Source: CAD feature listing. Evaluate the final solid. Frame: model axes, mm. A direction names the side the tool comes from. Round coordinates to 2 decimals unless told otherwise and drop trailing zeros. Write each loop counter-clockwise with the first axis right and the second up, starting at its lowest first coordinate (ties: lowest second). Pieces come first, ordered by that corner, then holes.
```python
from build123d import *

# Parameters (mm, degrees)
SKETCH1_R               = 4.7625
BOSS_EXTRUDE1_DEPTH     = 5.08
SKETCH2_W               = 5.08
SKETCH2_H               = 4.445
SKETCH3_R               = 1.27
CUT_EXTRUDE1_DEPTH      = 1
CUT_EXTRUDE1_DEPTH_BACK = 11.16


with BuildPart() as part:
    # Sketch1 → Boss-Extrude1 (new body, symmetric)
    with BuildSketch(Plane.XY):
        Circle(SKETCH1_R)
    extrude(amount=BOSS_EXTRUDE1_DEPTH, both=True)

    # Sketch2 → Cut-Revolve1 (revolve, cut)
    with BuildSketch(Plane(origin=(0, 0, 0), x_dir=(0, 0, -1), z_dir=(1, 0, 0)), mode=Mode.PRIVATE) as cut_revolve1_sk:
        with Locations((0, 4.7625)):
            Rectangle(SKETCH2_W, SKETCH2_H)
    revolve(cut_revolve1_sk.sketch.rotate(Axis((0, 0, 0), (0, 0, -1)), 180), axis=Axis((0, 0, 0), (0, 0, -1)), mode=Mode.SUBTRACT)  # turned: the seam where the file's is

    # Sketch3 → Cut-Extrude1 (cut, two sides)
    with BuildSketch(Plane.XY.offset(5.08)) as cut_extrude1_sk:
        Circle(SKETCH3_R)
    extrude(amount=CUT_EXTRUDE1_DEPTH, mode=Mode.SUBTRACT)
    extrude(cut_extrude1_sk.sketch, amount=-CUT_EXTRUDE1_DEPTH_BACK, mode=Mode.SUBTRACT)


solid = part.part
```
Q1. Line query: line 1 (Z direction, x = -1.5, y = 2.25); line 2 (Y direction, x = 0, z = 2.75); line 3 (X direction, y = -0.75, z = -4.25). Output: solid intervals per line, ascending.
Q2. Section query D-D, the plane x = -4. Output: boundary loops of the cut face in (y, z).
Q3. Section query A-A, the plane y = 0. Output: boundary loops of the cut face in (x, z), and give its area (3 significant figures).
Q4. Pin query (flat end, axial travel): P1, Ø4, axis at y = -0.5, z = 2, coming from the +X side; P2, Ø3, axis at x = -2, z = -3, coming from the -Y side; P3, Ø1, axis at x = 2, z = 0, coming from the -Y side; P4, Ø1.5, axis at y = -2, z = -3.5, coming from the +X side. Return the tip coordinate at first contact, or that it passes through.
Q5. Section query C-C, the plane z = -3.75. Output: boundary loops of the cut face in (x, y) (1 decimal).
Q6. Set-up query: faces 1 (the face through (-0.17, 1.26, 0.07)), 2 (the face through (2, 2, 2.54)). Return all of +Z, -Z, +X, -X, +Y, -Y with unobstructed straight access to the full face (end or side cutting, diameter ignored); none if empty.
Q7. Mould query, pull axis Z, two halves, no side actions, for faces 3 (the face through (-3.78, -2.9, -3.79)), 4 (the face through (1, 1.1, -5.08)), 5 (the face through (-2.52, 0.33, -0.04)). Classes: pulls with the +Z half, pulls with the -Z half, needs draft (parallel to the pull), parting line crosses it, or undercut.
Filled in:
1. line 1: z = -5.08 to -2.54, 2.54 to 5.08
1. line 2: y = -4.76 to -1.27, 1.27 to 4.76
1. line 3: x = -4.7 to -1.02, 1.02 to 4.7
2. outline: (-2.58, -5.08) - (2.58, -5.08) - (2.58, -2.54) - (-2.58, -2.54) - close; (-2.58, 2.54) - (2.58, 2.54) - (2.58, 5.08) - (-2.58, 5.08) - close
3. outline: (-4.76, -5.08) - (-1.27, -5.08) - (-1.27, 5.08) - (-4.76, 5.08) - (-4.76, 2.54) - (-2.54, 2.54) - (-2.54, -2.54) - (-4.76, -2.54) - close; (1.27, -5.08) - (4.76, -5.08) - (4.76, -2.54) - (2.54, -2.54) - (2.54, 2.54) - (4.76, 2.54) - (4.76, 5.08) - (1.27, 5.08) - close
3. area: 48.4 mm2
4. P1: stops at x = 4.76
4. P2: stops at y = -4.74
4. P3: stops at y = -2.05
4. P4: stops at x = 4.6
5. outline: circle Ø9.5 at (0, 0); hole circle Ø2.5 at (0, 0)
6. face 1: +Z, -Z
6. face 2: none
7. face 3: needs draft
7. face 4: pulls with the -Z half
7. face 5: undercut
